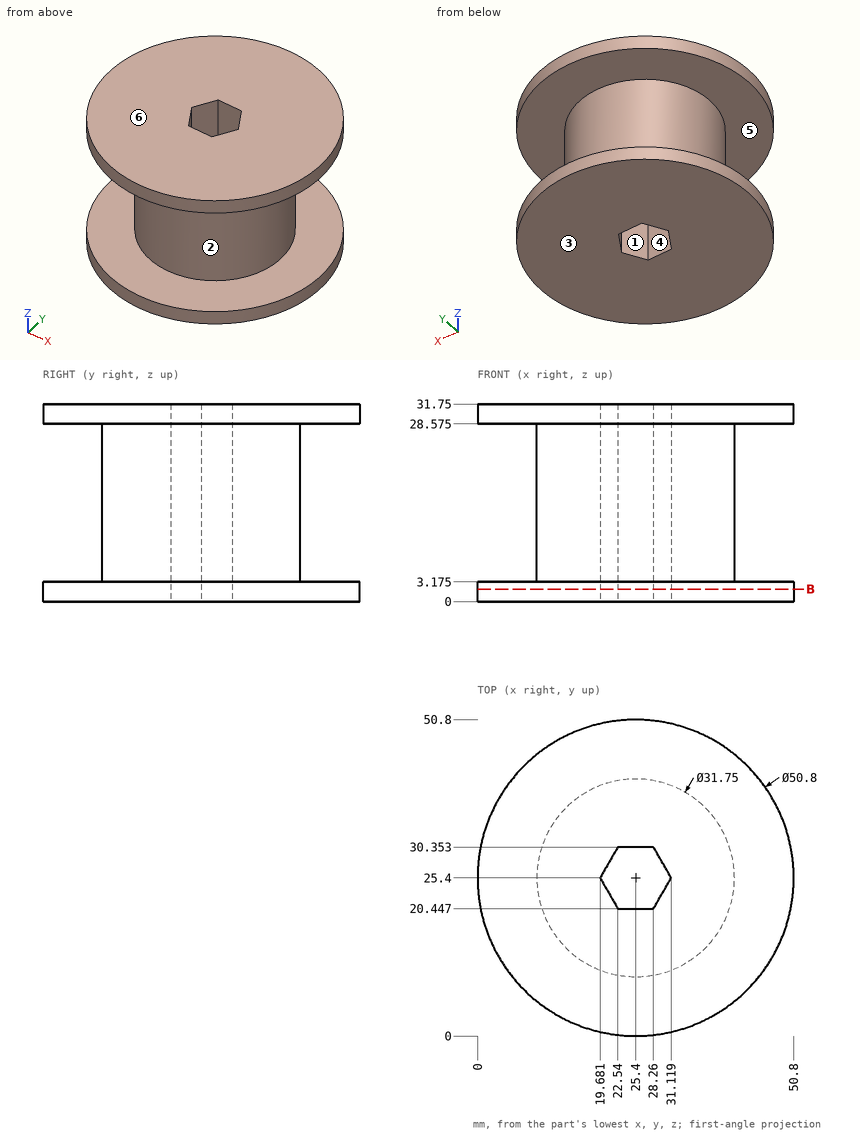
Could you check a few things on this drawing? It's one solid part, dimensions in mm from its lowest x, y, z. A direction names the side the tool comes from. Round coordinates to 2 decimals unless told otherwise and drop trailing zeros. Loops run counter-clockwise (first coordinate to the right, second up) from the corner with the lowest first, then second, coordinate; pieces in that order, holes last.
Q1. Please list where these lines run through material, in increasing order: L1, parallel to Y at x = 27.5, z = 15 (1 decimal); L2, parallel to Y at x = 30, z = 13 (1 decimal); L3, parallel to X at y = 22.5, z = 20.5 (1 decimal).
Q2. For P1, Ø6, axis at x = 30, y = 40.5, coming from the -Z side; P2, Ø4, axis at x = 18, z = 13.5, coming from the +Y side; P3, Ø1.5, axis at x = 28, z = 24, coming from the -Y side; P4, Ø3, axis at x = 26.5, z = 16.5, coming from the -Y side (3 decimals), each with a flat end and sliding along its axis, tell me the tip position at first contact or that it passes through.
Q3. I want a section at B-B (z = 2). Write out the boundary of the cut face in (x, y), and give its area (3 significant figures).
Q4. Thinking about a two-plate mould opening in Y: for the marked faces 1, 2 and 3, which applies, pulls with the +Y half, pulls with the -Y half, needs draft (parallel to the pull), parting line crosses it, or undercut?
Q5. On a 3-axis mill with a long thin cutter (end or side, diameter ignored), from which of +Z, -Z, +X, -X, +Y, -Y can I reach the whole of each face in a straight line? I mean the marked faces 4, 5 and 6. Say none if no direction works.
Answer below:
1. L1: y = 9.7 to 20.4, 30.4 to 41.1
1. L2: y = 10.2 to 23.5, 27.3 to 40.6
1. L3: x = 9.8 to 21.4, 29.4 to 41
2. P1: stops at z = 0
2. P2: stops at y = 40.33
2. P3: stops at y = 9.63
2. P4: stops at y = 9.525
3. outline: circle Ø50.8 at (25.4, 25.4); hole (19.68, 25.4) - (22.54, 20.45) - (28.26, 20.45) - (31.12, 25.4) - (28.26, 30.35) - (22.54, 30.35) - close
3. area: 1,940 mm2
4. face 1: undercut
4. face 2: parting line crosses it
4. face 3: needs draft
5. face 4: +Z, -Z
5. face 5: none
5. face 6: +Z, +X, -X, +Y, -Y
